Autodesk Inventor part; units mm, degrees
ref_plane "YZ Plane" through (0, 0, 0) normal (1, 0, 0) x (0, 1, 0)
ref_plane "XZ Plane" through (0, 0, 0) normal (0, 1, 0) x (-1, 0, 0)
ref_plane "XY Plane" through (0, 0, 0) normal (0, 0, 1) x (1, 0, 0)
sketch "Sketch1" plane through (0, 0, 0) normal (0, 0, 1) x (1, 0, 0)
  line L0 (-187.5, -150) -> (187.5, -150)
  line L1 (187.5, -150) -> (187.5, 150)
  line L2 (187.5, 150) -> (-187.5, 150)
  line L3 (-187.5, 150) -> (-187.5, -150)
  line L4 (-187.5, -150) -> (187.5, 150) construction
  line L5 (187.5, -150) -> (-187.5, 150) construction
  point P0 (0, 0)
  dimension "d0" = 375
  dimension "d1" = 300
extrude "Extrusion1" add sketch "Sketch1" along normal blind 6
sketch "Sketch6" plane through (0, 0, 0) normal (0, 0, -1) x (-1, 0, 0)
  line L0 (-187.5, 150) -> (-162.5, 150)
  line L1 (-162.5, 150) -> (-162.5, 125)
  line L2 (-162.5, 125) -> (-187.5, 125)
  line L3 (-187.5, 125) -> (-187.5, 150)
  line L4 (187.5, 150) -> (187.5, -150)
  line L5 (-187.5, 150) -> (187.5, 150)
  line L6 (-187.5, -150) -> (-187.5, 150)
  line L7 (-187.5, -35) -> (-162.5, -35)
  line L8 (-162.5, -35) -> (-162.5, -60)
  line L9 (-162.5, -60) -> (-187.5, -60)
  line L10 (-187.5, -60) -> (-187.5, -35)
  line L11 (187.5, -35) -> (162.5, -35)
  line L12 (162.5, -35) -> (162.5, -60)
  line L13 (162.5, -60) -> (187.5, -60)
  line L14 (187.5, -60) -> (187.5, -35)
  line L15 (62.5, 150) -> (37.5, 150)
  line L16 (37.5, 150) -> (37.5, 125)
  line L17 (37.5, 125) -> (62.5, 125)
  line L18 (62.5, 125) -> (62.5, 150)
  point P0 (0, 0)
  dimension "d22" = 25
  dimension "d25" = 160
  dimension "d26" = 200
extrude "Extrusion6" cut sketch "Sketch6" against normal through all
sketch "Sketch7" plane through (0, 0, 0) normal (0, 0, -1) x (-1, 0, 0)
  line L0 (-162.5, -60) -> (-187.5, -60)
  line L1 (-187.5, -150) -> (-187.5, -60)
  line L2 (187.5, -60) -> (187.5, -150)
  line L3 (187.5, -60) -> (162.5, -60)
  line L4 (62.5, 150) -> (187.5, 150)
  line L5 (37.5, 125) -> (37.5, 150)
  line L6 (-162.5, 150) -> (37.5, 150)
  line L7 (-162.5, 125) -> (-187.5, 125)
  line L8 (-187.5, -35) -> (-187.5, 125)
  line L9 (-162.5, 125) -> (-187.5, 125)
  line L10 (-187.5, 125) -> (-187.5, 91)
  line L11 (-187.5, 91) -> (-162.5, 91)
  line L12 (-162.5, 91) -> (-162.5, 125)
  line L13 (-162.5, 125) -> (-128.5, 125)
  line L14 (-128.5, 125) -> (-128.5, 150)
  line L15 (-128.5, 150) -> (-162.5, 150)
  line L16 (-162.5, 150) -> (-162.5, 125)
  line L17 (37.5, 125) -> (3.5, 125)
  line L18 (3.5, 125) -> (3.5, 150)
  line L19 (3.5, 150) -> (37.5, 150)
  line L20 (37.5, 150) -> (37.5, 125)
  line L21 (62.5, 125) -> (96.5, 125)
  line L22 (96.5, 125) -> (96.5, 150)
  line L23 (96.5, 150) -> (62.5, 150)
  line L24 (62.5, 150) -> (62.5, 125)
  line L25 (187.5, -35) -> (162.5, -35)
  line L26 (162.5, -35) -> (162.5, -1)
  line L27 (162.5, -1) -> (187.5, -1)
  line L28 (187.5, -1) -> (187.5, -35)
  line L29 (162.5, -60) -> (187.5, -60)
  line L30 (187.5, -60) -> (187.5, -94)
  line L31 (187.5, -94) -> (162.5, -94)
  line L32 (162.5, -94) -> (162.5, -60)
  line L33 (-162.5, -60) -> (-187.5, -60)
  line L34 (-187.5, -60) -> (-187.5, -94)
  line L35 (-187.5, -94) -> (-162.5, -94)
  line L36 (-162.5, -94) -> (-162.5, -60)
  line L37 (-162.5, -35) -> (-187.5, -35)
  line L38 (-187.5, -35) -> (-187.5, -1)
  line L39 (-187.5, -1) -> (-162.5, -1)
  line L40 (-162.5, -1) -> (-162.5, -35)
  point P0 (0, 0)
  dimension "d31" = 34
extrude "Extrusion7" cut sketch "Sketch7" against normal through all
sketch "Sketch8" plane through (0, 0, 6) normal (0, 0, 1) x (1, 0, 0)
  line L0 (187.5, -150) -> (187.5, 150)
  line L1 (128.5, 125) -> (128.5, 150)
  line L2 (187.5, 150) -> (-187.5, 150)
  line L3 (-187.5, -1) -> (-162.5, -1)
  line L4 (-162.5, -94) -> (-187.5, -94)
  line L5 (-187.5, -150) -> (187.5, -150)
  circle A0 centre (-175, 137.5) radius 2.7
  circle A1 centre (-175, 11.5) radius 2.7
  circle A2 centre (-175, -137.5) radius 2.7
  circle A3 centre (175, -137.5) radius 2.7
  circle A4 centre (175, 11.5) radius 2.7
  circle A5 centre (116, 137.5) radius 2.7
  line L6 (-175, -137.5) -> (-175, -94) construction
  point P0 (187.5, -1)
  point P1 (187.5, 91)
  point P2 (-96.5, 150)
  point P3 (0, 0)
  dimension "d32" = 12.5
  dimension "d33" = 12.5
  dimension "d34" = 12.5
  dimension "d35" = 12.5
  dimension "d36" = 12.5
  dimension "d37" = 5.4
extrude "Extrusion8" cut sketch "Sketch8" against normal blind 10
sketch "Sketch9" plane through (0, 0, 6) normal (0, 0, 1) x (1, 0, 0)
  line L0 (187.5, -150) -> (187.5, 150)
  line L1 (187.5, 150) -> (-187.5, 150)
  line L2 (-3.5, 125) -> (-96.5, 125)
  line L3 (187.5, -94) -> (162.5, -94)
  line L4 (5.5, 77.5) -> (5.5, 52.5) construction
  line L5 (3.35, 77.5) -> (3.35, 52.5)
  line L6 (7.65, 52.5) -> (7.65, 77.5)
  arc A0 (7.65, 77.5) -> (3.35, 77.5) centre (5.5, 77.5) ccw
  arc A1 (3.35, 52.5) -> (7.65, 52.5) centre (5.5, 52.5) ccw
  line L7 (5.5, -4.1) -> (5.5, 20.9) construction
  line L8 (3.35, -4.1) -> (3.35, 20.9)
  line L9 (7.65, 20.9) -> (7.65, -4.1)
  arc A2 (3.35, -4.1) -> (7.65, -4.1) centre (5.5, -4.1) ccw
  arc A3 (7.65, 20.9) -> (3.35, 20.9) centre (5.5, 20.9) ccw
  line L10 (119.5, 77.5) -> (119.5, 52.5) construction
  line L11 (117.35, 77.5) -> (117.35, 52.5)
  line L12 (121.65, 52.5) -> (121.65, 77.5)
  arc A4 (121.65, 77.5) -> (117.35, 77.5) centre (119.5, 77.5) ccw
  arc A5 (117.35, 52.5) -> (121.65, 52.5) centre (119.5, 52.5) ccw
  line L13 (119.5, 20.9) -> (119.5, -4.1) construction
  line L14 (117.35, 20.9) -> (117.35, -4.1)
  line L15 (121.65, -4.1) -> (121.65, 20.9)
  arc A6 (121.65, 20.9) -> (117.35, 20.9) centre (119.5, 20.9) ccw
  arc A7 (117.35, -4.1) -> (121.65, -4.1) centre (119.5, -4.1) ccw
  line L16 (-50, 125) -> (-50, -47.5) construction
  line L17 (-50, -47.5) -> (175, -47.5) construction
  line L18 (175, -47.5) -> (175, -94) construction
  line L19 (5.5, 8.4) -> (119.5, 8.4) construction
  line L20 (62.5, 8.4) -> (62.5, -47.5) construction
  point P0 (187.5, -1)
  point P1 (187.5, 91)
  point P2 (128.5, 150)
  point P3 (-3.5, 150)
  point P4 (0, 0)
  point P5 (5.5, 65)
  point P6 (119.5, 65)
  point P7 (-37.5, 125)
  point P8 (-62.5, 125)
  dimension "d40" = 114
  dimension "d41" = 2.15
  dimension "d42" = 56.6
  dimension "d43" = 25
  dimension "d44" = 85
extrude "Extrusion9" cut sketch "Sketch9" against normal blind 10
fillet "Fillet3" radius 6 12 edges at (187.5, -150, 3) (187.5, -94, 3) (187.5, -1, 3) (187.5, 91, 3) (162.5, 125, 3) (128.5, 150, 3) (-3.5, 150, 3) (-96.5, 150, 3) (-187.5, 150, 3) (-187.5, -94, 3) (-187.5, -150, 3) (-187.5, -1, 3)
equation "\"d33\" = d32"
equation "\"d34\" = d32"
equation "\"d35\" = d33"
equation "\"d36\" = d32"
properties part number "ProjectorPlateFront"
Could you check a few things on this model? Use its own coordinates, in mm. Give positions to 0.01 mm unless a question says otherwise; leave off trailing zeros. Write each loop counter-clockwise with the first axis right and the second up, starting at its lowest first coordinate (ties: lowest second). Pieces come first, ordered by that corner, then holes. Notation, with made-up numbers: (47, 36.5) - (84, 36.5) arc R26 cw to (84, 63.5) - close; hole circle Ø11 at (62.25, 12.5). An arc over 180 degrees is marked (long way). Use CSV: the item, a comma, the result in double quotes. Start each with the question number.
Item 1: I want a section at B-B, the plane x = -74. Please give me the cut outline in (y, z).
Item 2: I'm going to push flat-ended pins straight in: pin 1 (1.5 mm diameter, centred on y = 115, z = 1.5, fed in from +X); pin 2 (1.8 mm diameter, centred on x = 139, z = 3.5, fed in from +Y); pin 3 (1.8 mm diameter, centred on x = 171, z = 3.5, fed in from +Y). Where does each tip first touch, or does it pass through?
Item 3: I want a section at C-C, the plane y = -71. Please give me the cut outline in (x, z), then the cut area to 3 significant figures.
Item 4: I want a section at A-A, the plane z = 4.8. Give the number of separate pieces and of enclosed holes in the cut face, then the cut area to 3 significant figures.
Item 5: If I drill on line 1 along Y through (x, z) = (-175, 1.9); line 2 along X through (y, z) = (-4, 2.4); line 3 along X through (y, z) = (-137.5, 2.6), over which ranges is the centre line in solid material (lowest first)?
Findings:
1,outline,"(-150, 0) - (125, 0) - (125, 6) - (-150, 6) - close"
2,pin 1,"stops at x = 162.5"
2,pin 2,"stops at y = 125"
2,pin 3,"stops at y = 91"
3,outline,"(-162.5, 0) - (162.5, 0) - (162.5, 6) - (-162.5, 6) - close"
3,area,"1,950 mm2"
4,separate pieces,"1"
4,enclosed holes,"10"
4,area,"102,000 mm2"
5,line 1,"y = -150 to -140.2, -134.8 to -94, -1 to 8.8, 14.2 to 134.8, 140.2 to 150"
5,line 2,"x = -162.5 to 3.35, 7.65 to 117.35, 121.65 to 162.5"
5,line 3,"x = -187.5 to -177.7, -172.3 to 172.3, 177.7 to 187.5"
